Geometry check sheet. Reference: the model listing, model coordinates, mm. A direction names the side the tool comes from. Round coordinates to 2 decimals unless told otherwise and drop trailing zeros. Write each loop counter-clockwise with the first axis right and the second up, starting at its lowest first coordinate (ties: lowest second). Pieces come first, ordered by that corner, then holes. Notation, with made-up numbers: (-18, 83) -> (19, 83) arc R32 ccw to (19, 112) -> close; hole circle Ø2 at (-26, 54). An arc over 180 degrees is marked (long way). Return JSON: item names as keys, results as strings. Group by question number.
from build123d import *

# Parameters (mm, degrees)
SKETCH_1_W                 = 240
SKETCH_1_H                 = 100
EXTRUDE_1_DEPTH            = 6
SKETCH_2_R                 = 1.55
CUT_EXTRUDE_1_DEPTH        = 261.069221555
SKETCH_3_W                 = 60
SKETCH_3_H                 = 15
CUT_EXTRUDE_2_DEPTH        = 261.069221555
SKETCH_4_W                 = 30
SKETCH_4_H                 = 80
CUT_EXTRUDE_3_DEPTH        = 261.069221555
SKETCH_5_R                 = 3
CUT_EXTRUDE_4_DEPTH        = 3
EXTRUDE_2_DEPTH            = 240
EXTRUDE_3_DEPTH            = 5
PATTERN_LINEAR_1_COUNT     = 6
PATTERN_LINEAR_1_PITCH     = 20
PATTERN_LINEAR_1_COL_COUNT = 6
PATTERN_LINEAR_1_COL_PITCH = 20
FILLET_1_R                 = 5


with BuildPart() as part:
    # 草图1 → 凸台-拉伸1 (new body)
    with BuildSketch(Plane(origin=(0, 0, 0), x_dir=(0, 0, -1), z_dir=(1, 0, 0))):
        with Locations((120, -50)):
            Rectangle(SKETCH_1_W, SKETCH_1_H)
    extrude(amount=EXTRUDE_1_DEPTH)

    # 草图2 → 切除-拉伸1 (cut, through all)
    with BuildSketch(Plane(origin=(6, 0, 0), x_dir=(0, 0, -1), z_dir=(1, 0, 0))):
        with Locations((8, -54)):
            Circle(SKETCH_2_R)
        with Locations((45, -80)):
            Circle(SKETCH_2_R)
        with Locations((45, -54)):
            Circle(SKETCH_2_R)
        with Locations((8, -80)):
            Circle(SKETCH_2_R)
        with Locations(Location((232, -80, 0), (0, 0, 180))):
            Circle(SKETCH_2_R)
        with Locations(Location((195, -54, 0), (0, 0, 180))):
            Circle(SKETCH_2_R)
        with Locations(Location((195, -80, 0), (0, 0, 180))):
            Circle(SKETCH_2_R)
        with Locations(Location((232, -54, 0), (0, 0, 180))):
            Circle(SKETCH_2_R)
    extrude(amount=-CUT_EXTRUDE_1_DEPTH, mode=Mode.SUBTRACT)

    # 草图3 → 切除-拉伸2 (cut, through all)
    with BuildSketch(Plane(origin=(6, 0, 0), x_dir=(0, 0, -1), z_dir=(1, 0, 0))):
        with Locations((40, -27.5)):
            Rectangle(SKETCH_3_W, SKETCH_3_H)
        with Locations((200, -27.5)):
            Rectangle(SKETCH_3_W, SKETCH_3_H)
    extrude(amount=-CUT_EXTRUDE_2_DEPTH, mode=Mode.SUBTRACT)

    # 草图4 → 切除-拉伸3 (cut, through all)
    with BuildSketch(Plane(origin=(6, 0, 0), x_dir=(0, 0, -1), z_dir=(1, 0, 0))):
        with Locations((100, -50)):
            Rectangle(SKETCH_4_W, SKETCH_4_H)
        with Locations((140, -50)):
            Rectangle(SKETCH_4_W, SKETCH_4_H)
    extrude(amount=-CUT_EXTRUDE_3_DEPTH, mode=Mode.SUBTRACT)

    # 草图5 → 切除-拉伸4 (cut)
    with BuildSketch(Plane.ZY):
        with Locations((-195, -80)):
            Circle(SKETCH_5_R)
        with Locations((-232, -80)):
            Circle(SKETCH_5_R)
        with Locations((-195, -54)):
            Circle(SKETCH_5_R)
        with Locations((-232, -54)):
            Circle(SKETCH_5_R)
        with Locations((-45, -80)):
            Circle(SKETCH_5_R)
        with Locations((-8, -80)):
            Circle(SKETCH_5_R)
        with Locations((-8, -54)):
            Circle(SKETCH_5_R)
        with Locations((-45, -54)):
            Circle(SKETCH_5_R)
    extrude(amount=-CUT_EXTRUDE_4_DEPTH, mode=Mode.SUBTRACT)

    # 草图6 → 凸台-拉伸2 (add)
    with BuildSketch(Plane.XY):
        Polygon((6, 0), (0, 0), (0, 7.150521556), align=None)
    extrude(amount=-EXTRUDE_2_DEPTH)

    # 草图7 → 凸台-拉伸3 (add)
    with BuildSketch(Plane.XY.offset(-117.5)):
        Polygon((0, 7.150521556), (0, 13.150521556), (6, 2.75821671), (6, 0), align=None)
    extrude_3 = extrude(amount=-EXTRUDE_3_DEPTH)

    # 阵列(线性)1: 凸台-拉伸3 ×6
    with Locations(*[(0, 0, -i * PATTERN_LINEAR_1_PITCH) for i in range(1, PATTERN_LINEAR_1_COUNT)]):
        add(extrude_3)

    # 阵列(线性)1 col: 凸台-拉伸3 ×6
    with Locations(*[(0, 0, i * PATTERN_LINEAR_1_COL_PITCH) for i in range(1, PATTERN_LINEAR_1_COL_COUNT)]):
        add(extrude_3)

    # 圆角1
    fillet_1_edges = [part.edges().sort_by_distance(p)[0] for p in [
        (6, 2.75821671, -120),
        (6, 2.75821671, -100),
        (6, 2.75821671, -80),
        (6, 2.75821671, -60),
        (6, 2.75821671, -40),
        (6, 2.75821671, -20),
        (6, 2.75821671, -140),
        (6, 2.75821671, -160),
        (6, 2.75821671, -180),
        (6, 2.75821671, -200),
        (6, 2.75821671, -220),
    ]]
    fillet(fillet_1_edges, radius=FILLET_1_R)


solid = part.part
1) Mould release check, pull along Z, two halves, no side actions. Record for faces 5 (the face through (2.628, 8.599, -39.965)), 6 (the face through (3, 6, -17.5)), 7 (the face through (3, 6, -137.5)): +Z half, -Z half, draft (parallel to the pull), parting line (faces both ways), or undercut.
2) Tool access check on faces 1 (the face through (3, -51, -85)), 2 (the face through (1.48, -82.93, -45.65)), 3 (the face through (3, 6, -217.5)), 4 (the face through (2.958, 3.625, -231.128)). Record the directions out of +Z, -Z, +X, -X, +Y, -Y that give a thin tool (end or side, any length) a straight path to the whole face; none if there is none.
3) Sectioned sample at A-A on z = -187. Enter the section's corners in (x, y).
4) Sectioned sample at D-D on x = 4.25. State how many separate pieces and enclosed holes the cut face has, and give its area (3 significant figures).
5) Sectioned sample at B-B on y = -74. Enter the section's corners in (x, z), and give its area (3 significant figures).
6) Sectioned sample at C-C on z = -92. Enter the section's corners in (x, y), and give its area (3 significant figures).
7) Go/stop test with flat-tipped pins: P1, Ø3, axis at x = 2.5, z = -35, coming from the +Y side; P2, Ø2, axis at x = 2, z = -101, coming from the +Y side; P3, Ø1.8, axis at y = -52.5, z = -232, coming from the -X side. Record where each tip stops, or that it passes through.
8) Material ranges on probe 1 along Z at (x, y) = (0.5, -28); probe 2 along Z at (x, y) = (2.75, -68); probe 3 along Y at (x, z) = (1, -108), recorded low to high. Write a range as [from, to].
Evaluation:
{
 "1": {"face 5": "draft", "face 6": "+Z half", "face 7": "undercut"},
 "2": {"face 1": "+X, -X", "face 2": "-X", "face 3": "+X, +Y", "face 4": "-Z, +X, +Y"},
 "3": {"outline": "(0, -100) -> (6, -100) -> (6, -35) -> (0, -35) -> close; (0, -20) -> (6, -20) -> (6, 0) -> (0, 7.15) -> close"},
 "4": {"separate pieces": "1", "enclosed holes": "12", "area": "18,000 mm2"},
 "5": {"outline": "(0, -240) -> (6, -240) -> (6, -155) -> (0, -155) -> close; (0, -125) -> (6, -125) -> (6, -115) -> (0, -115) -> close; (0, -85) -> (6, -85) -> (6, 0) -> (0, 0) -> close", "area": "1,080 mm2"},
 "6": {"outline": "(0, -100) -> (6, -100) -> (6, -90) -> (0, -90) -> close; (0, -10) -> (6, -10) -> (6, 0) -> (0, 7.15) -> close", "area": "141 mm2"},
 "7": {"P1": "stops at y = 5.96", "P2": "stops at y = 11.42", "P3": "stops at x = 3"},
 "8": {"probe 1": "z = [-240, -230], [-170, -155], [-125, -115], [-85, -70], [-10, 0]", "probe 2": "z = [-240, -155], [-125, -115], [-85, 0]", "probe 3": "y = [-100, -90], [-10, 5.96]"}
}
